Input: part model. Units: mm. Frame: model coordinates. A direction names the side the tool comes from. Coordinates: 2 decimals unless noted, no trailing zeros. Loops run counter-clockwise (first coordinate to the right, second up) from the corner with the lowest first, then second, coordinate; pieces in that order, holes last. Notation, with made-up numbers: (63, 83) - (116, 83) arc R24 ccw to (116, 111) - close; hole circle Ø3 at (68.5, 7). An arc over 180 degrees is marked (long way). Answer as CSV lines item,"result". Start each with the question number.
```python
from build123d import *

# Parameters (mm, degrees)
BOSS_EXTRUDE1_DEPTH = 40
CUT_EXTRUDE1_DEPTH  = 20


with BuildPart() as part:
    # Sketch1 → Boss-Extrude1 (new body)
    with BuildSketch(Plane(origin=(0, 0, 0), x_dir=(1, 0, 0), z_dir=(0, 1, 0))):
        with BuildLine():
            Line((10, -5.773502692), (94.102760382, -54.330254038))
            Line((94.102760382, -54.330254038), (79.102760382, -80.311016151))
            Line((79.102760382, -80.311016151), (0, -34.641016151))
            Line((0, -34.641016151), (-79.102760382, -80.311016151))
            Line((-79.102760382, -80.311016151), (-94.102760382, -54.330254038))
            Line((-94.102760382, -54.330254038), (-10, -5.773502692))
            ThreePointArc((-10, -5.773502692), (0, -3.094010768), (10, -5.773502692))
        make_face()
    extrude(amount=BOSS_EXTRUDE1_DEPTH)

    # Sketch2 → Cut-Extrude1 (cut)
    with BuildSketch(Plane(origin=(0, 40, 0), x_dir=(1, 0, 0), z_dir=(0, 1, 0))):
        Polygon((-86.602760382, -67.320635095), (0, -17.320508076), (86.602760382, -67.320635095), (84.102760382, -71.650762114), (0, -23.094010768), (-84.102760382, -71.650762114), align=None)
    extrude(amount=-CUT_EXTRUDE1_DEPTH, mode=Mode.SUBTRACT)


solid = part.part
```
Item 1: Section query A-A, the plane y = 27. Output: boundary loops of the cut face in (x, z).
Item 2: Section query B-B, the plane y = 7. Output: boundary loops of the cut face in (x, z), and give its area (3 significant figures).
Item 3: Material intervals for probe 1 along X at (y, z) = (35, 66); probe 2 along X at (y, z) = (37, 31); probe 3 along X at (y, z) = (33.5, 33), sorted ascending.
Item 4: Section query C-C, the plane z = 38. Output: boundary loops of the cut face in (x, y).
Item 5: Set-up query: faces 4 (the flat face through (40.11, 19.72, 57.8)), 5 (the flat face through (51.46, 19.72, 29.71)), 6 (the flat face through (13, 20, 30)). Return all of +Z, -Z, +X, -X, +Y, -Y with unobstructed straight access to the full face (end or side cutting, diameter ignored); none if empty.
Item 6: Draft query along Z for faces 1 (the flat face through (-86.5, 19.7, 67.5)), 2 (the cylindrical face through (-0.147, 19.72, 3.095)), 3 (the flat face through (42.64, 30.14, 47.71)). Return one class per face: pulls with the +Z half, pulls with the -Z half, needs draft (parallel to the pull), parting line crosses it, or undercut.
Item 7: Contact query for flat-ended pins moving along their axis: P1, Ø1, axis at y = 7, z = 40.5, coming from the +X side; P2, Ø12, axis at x = -33.5, y = 12.5, coming from the -Z side; P3, Ø1.5, axis at y = 16, z = 32, coming from the -X side; P4, Ø4, axis at x = -43.5, z = 21.5, coming from the -Y side. Output: stop coordinate, or through.
Item 8: Section query D-D, the plane x = -43. Output: boundary loops of the cut face in (y, z), and give its area (3 significant figures).
Response values:
1,outline,"(-94.1, 54.33) - (-10, 5.77) arc R20 ccw to (10, 5.77) - (94.1, 54.33) - (86.6, 67.32) - (0, 17.32) - (-86.6, 67.32) - close; (-84.1, 71.65) - (0, 23.09) - (84.1, 71.65) - (79.1, 80.31) - (0, 34.64) - (-79.1, 80.31) - close"
2,outline,"(-94.1, 54.33) - (-10, 5.77) arc R20 ccw to (10, 5.77) - (94.1, 54.33) - (79.1, 80.31) - (0, 34.64) - (-79.1, 80.31) - close"
2,area,"5,980 mm²"
3,probe 1,"x = -87.37 to -84.32, -74.32 to -54.32, 54.32 to 74.32, 84.32 to 87.37"
3,probe 2,"x = -53.69 to -23.69, -13.69 to 13.69, 23.69 to 53.69"
3,probe 3,"x = -57.16 to -27.16, -17.16 to 17.16, 27.16 to 57.16"
4,outline,"(-65.82, 0) - (-5.82, 0) - (-5.82, 40) - (-25.82, 40) - (-25.82, 20) - (-35.82, 20) - (-35.82, 40) - (-65.82, 40) - close; (5.82, 0) - (65.82, 0) - (65.82, 40) - (35.82, 40) - (35.82, 20) - (25.82, 20) - (25.82, 40) - (5.82, 40) - close"
5,face 4,"+Z, +Y, -Y"
5,face 5,"-Z, +X, +Y, -Y"
5,face 6,"+Y"
6,face 1,"pulls with the +Z half"
6,face 2,"pulls with the -Z half"
6,face 3,"undercut"
7,P1,"stops at x = 71.01"
7,P2,"stops at z = 15.88"
7,P3,"stops at x = -56.72"
7,P4,"passes through"
8,outline,"(0, 24.83) - (40, 24.83) - (40, 42.15) - (20, 42.15) - (20, 47.92) - (40, 47.92) - (40, 59.47) - (0, 59.47) - close"
8,area,"1,270 mm²"
